```python
from build123d import *

# Parameters (mm, degrees)
F0_W     = 300.2
F0_H     = 150.2
F1_DEPTH = 5
F2_W     = 4.9
F2_H     = 4.9
F2_W_2   = 40.1
F2_H_2   = 40.1
F2_H_3   = 39.8
F2_W_3   = 39.8
F3_DEPTH = 5


with BuildPart() as f1:
    # F0 (on Front) → F1 (new body)
    with BuildSketch(Plane.XZ):
        Rectangle(F0_W, F0_H)
    extrude(amount=F1_DEPTH)

    # F2 (on face) → F3 (cut, through all)
    with BuildSketch(Plane.XZ.offset(5)):
        with Locations((-147.65, 72.65)):
            Rectangle(F2_W, F2_H)
        with Locations((-125.15, 72.65)):
            Rectangle(F2_W_2, F2_H)
        with Locations((-147.65, 50.15)):
            Rectangle(F2_W, F2_H_2)
        with Locations((-147.65, 0)):
            Rectangle(F2_W, F2_H_3)
        with Locations((-147.65, -50.15)):
            Rectangle(F2_W, F2_H_2)
        with Locations((-147.65, -72.65)):
            Rectangle(F2_W, F2_H)
        with Locations((-125.15, -72.65)):
            Rectangle(F2_W_2, F2_H)
        with Locations((-75, 72.65)):
            Rectangle(F2_W_3, F2_H)
        with Locations((-25, 72.65)):
            Rectangle(F2_W_3, F2_H)
        with Locations((25, 72.65)):
            Rectangle(F2_W_3, F2_H)
        with Locations((75, 72.65)):
            Rectangle(F2_W_3, F2_H)
        with Locations((147.65, 72.65)):
            Rectangle(F2_W, F2_H)
        with Locations((125.15, 72.65)):
            Rectangle(F2_W_2, F2_H)
        with Locations((147.65, 50.15)):
            Rectangle(F2_W, F2_H_2)
        with Locations((25, -72.65)):
            Rectangle(F2_W_3, F2_H)
        with Locations((-25, -72.65)):
            Rectangle(F2_W_3, F2_H)
        with Locations((-75, -72.65)):
            Rectangle(F2_W_3, F2_H)
        with Locations((125.15, -72.65)):
            Rectangle(F2_W_2, F2_H)
        with Locations((147.65, -72.65)):
            Rectangle(F2_W, F2_H)
        with Locations((147.65, -50.15)):
            Rectangle(F2_W, F2_H_2)
        with Locations((75, -72.65)):
            Rectangle(F2_W_3, F2_H)
        with Locations((147.65, 0)):
            Rectangle(F2_W, F2_H_3)
    extrude(amount=-F3_DEPTH, mode=Mode.SUBTRACT)


solid = f1.part
```
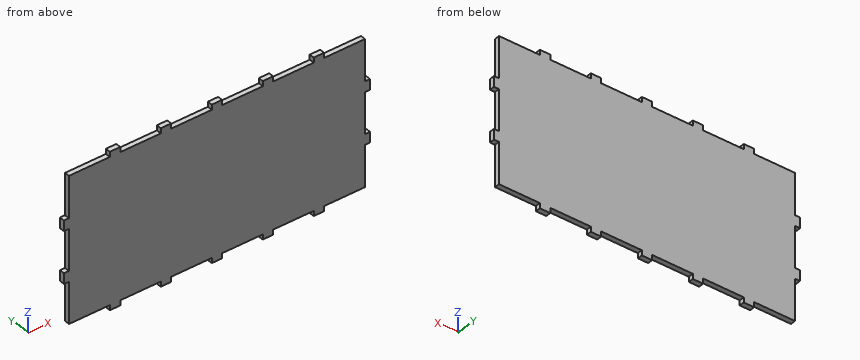
CAD build for the part. Positions are in the model's coordinates, mm. Round coordinates to 2 decimals unless told otherwise and drop trailing zeros. Write each loop counter-clockwise with the first axis right and the second up, starting at its lowest first coordinate (ties: lowest second). Pieces come first, ordered by that corner, then holes.
Item 1: Drop flat-ended pins along their axis: pin 1 Ø2.5 at (x, y) = (30, -2) entering from -Z; pin 2 Ø2.5 at (y, z) = (-3, -74) entering from -X; pin 3 Ø1.5 at (x, y) = (-147.5, -3) entering from -Z. Give the stop position or say it passes through.
Filled in:
pin 1: stops at z = -70.2
pin 2: stops at x = -105.1
pin 3: stops at z = -30.1
Item 2: Band-saw the part on B-B on z = -50. Write the cut outline in (x, y).
Filled in:
outline: (-145.2, -5) - (145.2, -5) - (145.2, 0) - (-145.2, 0) - close
Item 3: Band-saw the part on A-A on x = -116.5. Write the cut outline in (y, z), then the cut area to 3 significant figures.
Filled in:
outline: (-5, -70.2) - (0, -70.2) - (0, 70.2) - (-5, 70.2) - close
area: 702 mm2
Item 4: Drill centre lines: L1, parallel to X at y = -2.45, z = 19.5; L2, parallel to Z at x = 74.5, y = -3.6. Where is each one in solid material? Low to high.
Filled in:
L1: x = -145.2 to 145.2
L2: z = -70.2 to 70.2
